from build123d import *

# Parameters (mm, degrees)
PAD_DEPTH           = 50
SKETCH001_W         = 170
SKETCH001_H         = 160
PAD001_DEPTH        = 20
FILLET_R            = 5
PAD002_DEPTH        = 70
FILLET001_R         = 5
POCKET_DEPTH        = 70
POCKET001_DEPTH     = 70
POCKET002_DEPTH     = 70
HOLE_D              = 6.6
HOLE_CBORE_D        = 11
HOLE_CBORE_DEPTH    = 1.8
HOLE001_D           = 6.6
HOLE001_CBORE_D     = 11
HOLE001_CBORE_DEPTH = 1.8
HOLE002_D           = 6.6
HOLE002_CBORE_D     = 11
HOLE002_CBORE_DEPTH = 1.8


with BuildPart() as part:
    # Sketch → Pad (new body)
    with BuildSketch(Plane.XZ):
        with BuildLine():
            Line((0, 0), (0, 40))
            ThreePointArc((10, 50), (2.9289321881, 47.0710678119), (0, 40))
            Line((10, 50), (110, 50))
            ThreePointArc((120, 39.9999996097), (117.0710679499, 47.0710676739), (110, 50))
            Line((120, 39.9999996097), (119.9999988291, 9.9999996097))
            ThreePointArc((109.999957026, 1e-10), (117.0710517233, 2.9289172705), (119.9999988291, 9.9999996097))
            Line((109.999957026, 1e-10), (60, 0))
            ThreePointArc((60, 0), (52.9289320942, -2.9289322821), (50, -10.0000002657))
            Line((50, -10.0000002657), (50, -59.9999999242))
            ThreePointArc((40, -69.9999999242), (47.0710678119, -67.0710677361), (50, -59.9999999242))
            Line((40, -69.9999999242), (10, -69.9999999242))
            ThreePointArc((0, -60), (2.9289322149, -67.0710677629), (10, -69.9999999242))
            Line((0, -60), (0, 0))
        make_face()
    extrude(amount=PAD_DEPTH)

    # Sketch001 → Pad001 (join)
    with BuildSketch(Plane.XZ.offset(50)):
        with Locations((65, -10)):
            Rectangle(SKETCH001_W, SKETCH001_H)
    extrude(amount=PAD001_DEPTH)

    # Fillet
    fillet_edges = [part.edges().sort_by_distance(p)[0] for p in [
        (-20, -60, 70),
        (-20, -60, -90),
        (150, -60, 70),
        (65, -50, 70),
        (-20, -50, -10),
        (150, -50, -10),
        (150, -60, -90),
        (65, -50, -90),
    ]]
    fillet(fillet_edges, radius=FILLET_R)

    # Sketch002 → Pad002 (join)
    with BuildSketch(Plane(origin=(0, 0, 0), x_dir=(1, 0, 0), z_dir=(0, 1, 0))):
        with BuildLine():
            ThreePointArc((0, -40.0000140922), (2.9289421532, -47.0710777769), (10.0000140931, -50))
            Line((10.0000140931, -50), (40, -50))
            ThreePointArc((40, -50), (47.0710678169, -47.0710678069), (50, -39.9999999859))
            Line((50, -9.9999998015), (50, -39.9999999859))
            ThreePointArc((50, -9.9999998015), (47.0710677417, -2.928932118), (40, 0))
            Line((10, -1e-10), (40, 0))
            ThreePointArc((10, -1e-10), (2.9288998762, -2.9289222234), (-4.22766e-05, -10.0000140922))
            Line((0, -40.0000140922), (-4.22766e-05, -10.0000140922))
        make_face()
    extrude(amount=PAD002_DEPTH)

    # Fillet001
    fillet001_edges = [part.edges().sort_by_distance(p)[0] for p in [
        (47.071068, 70, 2.928932),
    ]]
    fillet(fillet001_edges, radius=FILLET001_R)

    # Sketch003 → Pocket (cut)
    with BuildSketch(Plane(origin=(119.9999984388, 0, -4.6837e-06), x_dir=(3.9e-08, 0, 1), z_dir=(1, 0, -3.9e-08))):
        with BuildLine():
            Line((6.0004431316, 5), (44.0000020269, 5))
            ThreePointArc((44.0000020269, 5), (44.7071074978, 5.2928939354), (45, 6))
            Line((45, 6), (45, 44))
            ThreePointArc((45, 44), (44.7071067529, 44.7071067294), (44, 44.9999999199))
            Line((44, 44.9999999199), (6, 44.9999999199))
            ThreePointArc((6, 44.9999999199), (5.292893205, 44.7071066873), (5, 43.999999881))
            Line((5, 43.999999881), (5, 5.999999881))
            ThreePointArc((5, 5.999999881), (5.2930499143, 5.2927364599), (6.0004431316, 5))
        make_face()
    extrude(amount=-POCKET_DEPTH, mode=Mode.SUBTRACT)

    # Sketch004 → Pocket001 (cut)
    with BuildSketch(Plane(origin=(0, 0, -69.9999999242), x_dir=(1, 0, 0), z_dir=(0, 0, -1))):
        with BuildLine():
            Line((5.9999900445, 5), (43.9999900445, 5))
            ThreePointArc((43.9999900445, 5), (44.7071032614, 5.292889699), (45, 6))
            Line((45, 6), (45, 43.9999998885))
            ThreePointArc((45, 43.9999998885), (44.7071068206, 44.7071067418), (44, 45))
            Line((44, 45), (6, 45))
            ThreePointArc((6, 45), (5.2928932188, 44.7071067812), (5, 44))
            Line((5, 44), (5, 6))
            ThreePointArc((5, 6), (5.292889699, 5.2928967386), (5.9999900445, 5))
        make_face()
    extrude(amount=-POCKET001_DEPTH, mode=Mode.SUBTRACT)

    # Sketch005 → Pocket002 (cut)
    with BuildSketch(Plane(origin=(0, 70, 0), x_dir=(1, 0, 0), z_dir=(0, 1, 0))):
        with BuildLine():
            Line((6, -4.9999917709), (44, -4.9999917709))
            ThreePointArc((45, -6), (44.7071096906, -5.2928878992), (44, -4.9999917709))
            Line((45, -6), (45, -44))
            ThreePointArc((44, -45), (44.7071067812, -44.7071067812), (45, -44))
            Line((44, -45), (6, -45))
            ThreePointArc((5, -44), (5.2928932224, -44.7071067747), (6, -44.9999999899))
            Line((5, -44), (5, -6))
            ThreePointArc((6, -4.9999917709), (5.2928903094, -5.2928878992), (5, -6))
        make_face()
    extrude(amount=-POCKET002_DEPTH, mode=Mode.SUBTRACT)

    # Hole (through all)
    with Locations(Plane(origin=(0, 0, 50), x_dir=(-1, 0, 0), z_dir=(0, 0, 1))):
        with Locations((-75, 25), (-100, 25)):
            CounterBoreHole(HOLE_D / 2, HOLE_CBORE_D / 2, HOLE_CBORE_DEPTH)

    # Hole001 (through all)
    with Locations(Plane(origin=(0, 0, 0), x_dir=(0, 0, -1), z_dir=(-1, 0, 0))):
        with Locations((50, 25), (25, 25)):
            CounterBoreHole(HOLE001_D / 2, HOLE001_CBORE_D / 2, HOLE001_CBORE_DEPTH)

    # Hole002 (through all)
    with Locations(Plane(origin=(-5.63689e-05, 0, 1e-10), x_dir=(-1.4092e-06, 0, -1), z_dir=(-1, 0, 1.4092e-06))):
        with Locations((-25, -25), (-25, -50)):
            CounterBoreHole(HOLE002_D / 2, HOLE002_CBORE_D / 2, HOLE002_CBORE_DEPTH)


solid = part.part
Build history of the part. All positions in model axes, mm. A direction names the side the tool comes from. Coordinates: 2 decimals unless noted, no trailing zeros. Order: outer loops, then holes, each group sorted by start corner. A loop starts at its lowest first (then second) coordinate and runs counter-clockwise, first axis right, second up. Notation, with made-up numbers: M -10,30 L 8,30 A20 ccw 8,69 Z; hole C -11.75,-11.75 d9. An arc over 180 degrees is marked long. One line per question, with ' | ' between items. Start each with the question number.
Q1. Saw through at D-D (y = -25). Count the separate pieces of the cut face and the enclosed holes in it, then the cut area to 3 significant figures.
Q2. Saw through at C-C (y = 50). List the corners of the cut face in (x, z).
Q3. Flat gauge pins, fed straight in: pin 1 Ø12 at (x, y) = (62.5, -41) entering from -Z; pin 2 Ø24 at (y, z) = (22, 29.5) entering from +X; pin 3 Ø10 at (x, y) = (48.5, 20.5) entering from -Z; pin 4 Ø4 at (y, z) = (25, 25) entering from -X. Where does each tip first touch, or does it go through?
Q4. 3-axis set-ups, long thin cutter, end or side, ignore diameter. For faces 4 (the face through (71, -25, 48.2)), 5 (the face through (3.01, 32.04, 2.85)), 6 (the face through (0.887, -25.242, -44.505)), 7 (the face through (45, 35, 25)), 8 (the face through (85, -25, 5)): which of +Z, -Z, +X, -X, +Y, -Y reach the whole face in a straight line?
Q5. Two-plate mould, pull along X, no slides. Class faces 1 (the face through (99.28, -21.78, 46.58)), 2 (the face through (116, -25, 48)), 3 (the face through (47.54, 46.73, 24.57)): +X half, -X half, draft (parallel to the pull), parting line (faces both ways), or undercut.
Q6. Saw through at B-B (x = 84). List the corners of the cut face in (y, z).
Q7. Probe L1, parallel to Y at x = 93.5, z = 7; L2, parallel to Y at x = 100, z = 47; L3, parallel to Z at x = 91, y = -33.5. List the from-to ranges inside material, lowest first. Write a range as from..to.
Check values:
1) separate pieces: 9 | enclosed holes: 0 | area: 3,530 mm2
2) outline: M 0,10 A10 ccw 10,0 L 40,0 A10 ccw 50,10 L 50,21.7 L 45,21.7 L 45,6 A1 cw 44,5 L 6,5 A1 cw 5,6 L 5,21.7 L 1.8,21.7 L 1.8,19.5 L 0,19.5 Z; M 0,30.5 L 1.8,30.5 L 1.8,28.3 L 5,28.3 L 5,44 A1 cw 6,45 L 44,45 A1 cw 45,44 L 45,28.3 L 50,28.3 L 50,40 A10 ccw 40,50 L 10,50 A10 ccw 0,40 Z
3) pin 1: stops at z = -0.63 | pin 2: stops at x = 50 | pin 3: stops at z = 0.63 | pin 4: passes through
4) face 4: +Z | face 5: -Z, -X, +Y | face 6: -X | face 7: +Y | face 8: +X
5) face 1: undercut | face 2: +X half | face 3: draft
6) outline: M -70,-90 L -55,-90 A5 ccw -50,-85 L -50,0 L 0,0 L 0,50 L -50,50 L -50,65 A5 ccw -55,70 L -70,70 Z; hole M -45,6 A1 ccw -44,5 L -6,5 A1 ccw -5,6 L -5,44 A1 ccw -6,45 L -44,45 A1 ccw -45,44 Z
7) L1: y = -70..-45, -5..0 | L2: y = -70..-28.3, -21.7..0 | L3: z = 0..5, 45..50
